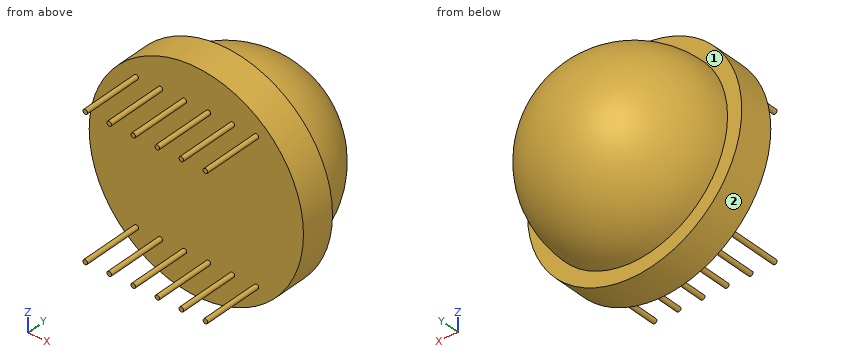
from build123d import *

# Parameters (mm, degrees)
SKETCH2_R           = 0.25
BOSS_EXTRUDE1_DEPTH = 6.5


with BuildPart() as part:
    # Sketch1 → Revolve1 (revolve)
    with BuildSketch(Plane.XY):
        with BuildLine():
            Line((0, 10.055), (0, 0))
            Line((0, 0), (0, -3.7))
            Line((0, -3.7), (-11.595, -3.7))
            Line((-11.595, -3.7), (-11.595, 0))
            Line((-11.595, 0), (-10.055, 0))
            ThreePointArc((-10.055, 0), (-7.109958685, 7.109958685), (0, 10.055))
        make_face()
    revolve(axis=Axis((0, 10.055, 0), (0, -1, 0)))

    # Sketch2 → Boss-Extrude1 (add)
    with BuildSketch(Plane.XZ.offset(3.7)):
        with Locations((-6.505, 7.605)):
            Circle(SKETCH2_R)
        with Locations((-3.903, 7.605)):
            Circle(SKETCH2_R)
        with Locations((-1.301, 7.605)):
            Circle(SKETCH2_R)
        with Locations((1.301, 7.605)):
            Circle(SKETCH2_R)
        with Locations((3.903, 7.605)):
            Circle(SKETCH2_R)
        with Locations((6.505, 7.605)):
            Circle(SKETCH2_R)
        with Locations((-3.903, -7.605)):
            Circle(SKETCH2_R)
        with Locations((-1.301, -7.605)):
            Circle(SKETCH2_R)
        with Locations((1.301, -7.605)):
            Circle(SKETCH2_R)
        with Locations((3.903, -7.605)):
            Circle(SKETCH2_R)
        with Locations((6.505, -7.605)):
            Circle(SKETCH2_R)
        with Locations((-6.505, -7.605)):
            Circle(SKETCH2_R)
    extrude(amount=BOSS_EXTRUDE1_DEPTH)


solid = part.part
The model under review builds one solid part; all positions refer to its coordinate system, in mm. Face numbers are marked on the shaded views. A direction names the side the tool comes from. Give positions to 0.01 mm unless a question says otherwise; leave off trailing zeros. Loops run counter-clockwise (first coordinate to the right, second up) from the corner with the lowest first, then second, coordinate; pieces in that order, holes last. Notation, with made-up numbers: (62, -35.75) -> (97, -35.75) arc R29 ccw to (97, 1.25) -> close; hole circle Ø11 at (-10.75, 21). An arc over 180 degrees is marked (long way). Write each question's results on one line, items separated by ' | '.
1) Take a section at A-A, the plane y = -7.25. Count the separate pieces of the cut face and the enclosed holes in it, plus the area to 3 significant figures.
Conclusion:
separate pieces: 12 | enclosed holes: 0 | area: 2.36 mm^2
2) Take a section at C-C, the plane x = 3. Give the boundary of the cut face in (y, z), plus the area to 3 significant figures.
Conclusion:
outline: (-3.7, -11.2) -> (0, -11.2) -> (0, -9.6) arc R9.6 ccw to (0, 9.6) -> (0, 11.2) -> (-3.7, 11.2) -> close | area: 228 mm^2
3) Tool access review of the marked faces 1 and 2: name each direction out of +Z, -Z, +X, -X, +Y, -Y from which nothing blocks a thin tool from reaching the whole face with its end or side.
Conclusion:
face 1: +Y | face 2: +Y, -Y
4) Insertion check: pin 1 Ø3 at (x, y) = (-5, -2.5) entering from -Z; pin 2 Ø5 at (y, z) = (4, 3.5) entering from -X; pin 3 Ø8 at (x, z) = (-5, 2.5) entering from +Y; pin 4 Ø1.5 at (x, z) = (9, 9) entering from +Y. Each pin has a flat end and moves straight along its axis. Give the tip position at first contact, or say it passes through.
Conclusion:
pin 1: stops at z = -11.05 | pin 2: stops at x = -9.65 | pin 3: stops at y = 9.93 | pin 4: passes through
5) For line 1 along Y through (x, z) = (2.25, 10.25); line 2 along Z through (x, y) = (-1, 4.25); line 3 along X through (y, z) = (2, 2), list the stretches that pass through material, from the lowest coordinate up. Write a range as from..to.
Conclusion:
line 1: y = -3.7..0 | line 2: z = -9.06..9.06 | line 3: x = -9.65..9.65
6) Take a section at D-D, the plane y = 1.5. Give the boundary of the cut face in (x, z).
Conclusion:
outline: circle Ø19.88 at (0, 0)
7) Take a section at B-B, the plane z = 0. Give the boundary of the cut face in (x, y) (3 decimals), plus the area to 3 significant figures.
Conclusion:
outline: (-11.595, -3.7) -> (11.595, -3.7) -> (11.595, 0) -> (10.055, 0) arc R10.055 ccw to (-10.055, 0) -> (-11.595, 0) -> close | area: 245 mm^2
